Read the model definition and answer for the solid it produces. Units are mm, in the model's axes. Face numbers are marked on the shaded views. A direction names the side the tool comes from. Coordinates: 2 decimals unless noted, no trailing zeros. Write each loop counter-clockwise with the first axis right and the second up, starting at its lowest first coordinate (ties: lowest second). Pieces come first, ordered by that corner, then holes.
1) The part is cut by section C-C (y = 20.5). Determine the outline of the cut face in (x, z), then the cut area to 3 significant figures.
2) The part is cut by section D-D (x = 14). Determine the outline of the cut face in (y, z).
3) Each of these flat-tipped pins is pushed along its axis until it touches: pin 1 Ø0.7 at (y, z) = (40.5, 13) entering from +X; pin 2 Ø0.5 at (x, z) = (-20, 5) entering from +Y; pin 3 Ø3.5 at (x, z) = (1, -8) entering from -Y. Where does it stop, or does it pass through?
4) Find the intervals of material crossed by line 1 (X direction, y = 37, z = 20); line 2 (Z direction, x = -14.5, y = 7.5); line 3 (X direction, y = 20, z = 20.5), in increasing order.
5) Which of the six approach directions +Z, -Z, +X, -X, +Y, -Y give full straight-line access (tool end or side, diameter ignored) to the marked faces 1, 2, 3, 4 and 5?
6) The part is cut by section A-A (x = 0). Determine the outline of the cut face in (y, z).
7) Determine the mould class of the marked faces 6, 7 and 8 for opening direction X: +X half, -X half, draft (parallel to the pull), parting line (faces both ways), or undercut.
8) The part is cut by section B-B (z = 3.5). Determine the outline of the cut face in (x, y).
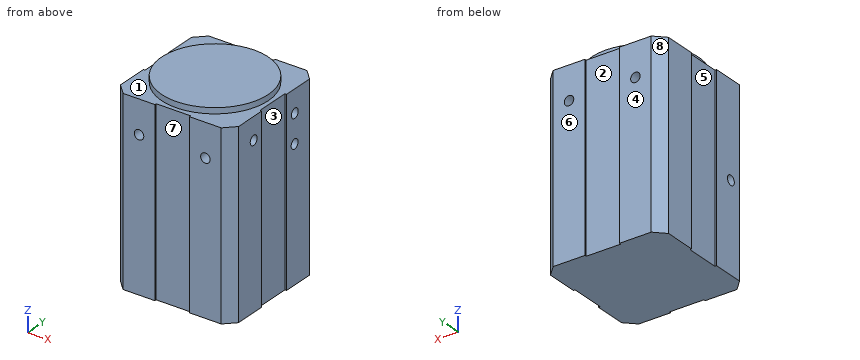
from build123d import *

# Parameters (mm, degrees)
SKETCH_1_W                       = 41
SKETCH_1_H                       = 63
EXTRUDE_1_DEPTH                  = 41
HOLE_WIZARD_M4_1_AT_2_COUNT      = 2
HOLE_WIZARD_M4_1_AT_2_PITCH      = 23
CHAMFER_1_SIZE                   = 3.5
CUT_EXTRUDE_1_REACH              = 79.912
SKETCH_4_W                       = 12
SKETCH_4_H                       = 0.6
SKETCH_4_W_2                     = 0.6
SKETCH_4_H_2                     = 12
SKETCH_5_R                       = 18.5
EXTRUDE_2_DEPTH                  = 2
HOLE_WIZARD_M4_3_D               = 3.3
HOLE_WIZARD_M4_3_DEPTH           = 10.1
HOLE_WIZARD_M4_3_TIP             = 0.991420021
HOLE_WIZARD_M4_3_ON_FACE_2_D     = 3.3
HOLE_WIZARD_M4_3_ON_FACE_2_DEPTH = 10.1
HOLE_WIZARD_M4_3_ON_FACE_2_TIP   = 0.991420021


with BuildPart() as part:
    # 草图1 → 凸台-拉伸1 (new body)
    with BuildSketch(Plane(origin=(0, 0, 0), x_dir=(1, 0, 0), z_dir=(0, 1, 0))):
        Rectangle(SKETCH_1_W, SKETCH_1_H)
    extrude(amount=EXTRUDE_1_DEPTH)

    # 草图3 → M4 螺纹孔1 (revolve, cut)
    with BuildSketch(Plane(origin=(-11.5, 41, 20), x_dir=(0, 0, 1), z_dir=(1, 0, 0))):
        Polygon((0, 0), (0, 6.991420021), (1.65, 6), (1.65, 0), align=None)
    hole_wizard_m4_1 = revolve(axis=Axis((-11.5, 47.35, 20), (0, -1, 0)), mode=Mode.SUBTRACT)

    # M4 螺纹孔1 at 2: M4 螺纹孔1 ×2
    with Locations(*[(i * HOLE_WIZARD_M4_1_AT_2_PITCH, 0, 0) for i in range(1, HOLE_WIZARD_M4_1_AT_2_COUNT)]):
        add(hole_wizard_m4_1, mode=Mode.SUBTRACT)

    # 镜向1: M4 螺纹孔1 across plane
    add(hole_wizard_m4_1.mirror(Plane.ZX.offset(20.5)), mode=Mode.SUBTRACT)

    # 镜向1 copy 1 sketch → 镜向1 copy 1 (revolve, cut)
    with BuildSketch(Plane(origin=(11.5, 0, 20), x_dir=(0, 0, 1), z_dir=(1, 0, 0))):
        Polygon((0, 0), (0, -6.991420021), (1.65, -6), (1.65, 0), align=None)
    revolve(axis=Axis((11.5, -6.35, 20), (0, -1, 0)), mode=Mode.SUBTRACT)

    # 倒角1
    chamfer_1_edges = [part.edges().sort_by_distance(p)[0] for p in [
        (-20.5, 41, 0),
        (20.5, 41, 0),
        (-20.5, 0, 0),
        (20.5, 0, 0),
    ]]
    chamfer(chamfer_1_edges, length=CHAMFER_1_SIZE)

    # 草图4 → 切除-拉伸1 (cut, up to next)
    with BuildSketch(Plane.XY.offset(31.5), mode=Mode.PRIVATE) as cut_extrude_1_sk1:
        with Locations((0, 40.7)):
            Rectangle(SKETCH_4_W, SKETCH_4_H)
    cut_extrude_1_tool1 = extrude(cut_extrude_1_sk1.sketch, amount=-CUT_EXTRUDE_1_REACH, mode=Mode.PRIVATE) & part.part
    # 草图4 → 切除-拉伸1 (cut, up to next)
    with BuildSketch(Plane.XY.offset(31.5), mode=Mode.PRIVATE) as cut_extrude_1_sk2:
        with Locations((20.2, 20.5)):
            Rectangle(SKETCH_4_W_2, SKETCH_4_H_2)
    cut_extrude_1_tool2 = extrude(cut_extrude_1_sk2.sketch, amount=-CUT_EXTRUDE_1_REACH, mode=Mode.PRIVATE) & part.part
    # 草图4 → 切除-拉伸1 (cut, up to next)
    with BuildSketch(Plane.XY.offset(31.5), mode=Mode.PRIVATE) as cut_extrude_1_sk3:
        with Locations((0, 0.3)):
            Rectangle(SKETCH_4_W, SKETCH_4_H)
    cut_extrude_1_tool3 = extrude(cut_extrude_1_sk3.sketch, amount=-CUT_EXTRUDE_1_REACH, mode=Mode.PRIVATE) & part.part
    # 草图4 → 切除-拉伸1 (cut, up to next)
    with BuildSketch(Plane.XY.offset(31.5), mode=Mode.PRIVATE) as cut_extrude_1_sk4:
        with Locations((-20.2, 20.5)):
            Rectangle(SKETCH_4_W_2, SKETCH_4_H_2)
    cut_extrude_1_tool4 = extrude(cut_extrude_1_sk4.sketch, amount=-CUT_EXTRUDE_1_REACH, mode=Mode.PRIVATE) & part.part
    add(cut_extrude_1_tool1.solids().sort_by_distance((0, 40.7, 31.5))[0], mode=Mode.SUBTRACT)
    add(cut_extrude_1_tool2.solids().sort_by_distance((20.2, 20.5, 31.5))[0], mode=Mode.SUBTRACT)
    add(cut_extrude_1_tool3.solids().sort_by_distance((0, 0.3, 31.5))[0], mode=Mode.SUBTRACT)
    add(cut_extrude_1_tool4.solids().sort_by_distance((-20.2, 20.5, 31.5))[0], mode=Mode.SUBTRACT)

    # 草图5 → 凸台-拉伸2 (add)
    with BuildSketch(Plane.XY.offset(31.5)):
        with Locations((0, 20.5)):
            Circle(SKETCH_5_R)
    extrude(amount=EXTRUDE_2_DEPTH)

    # M4 螺纹孔3
    with Locations(Plane(origin=(20.5, 30.405354364, 23.651006077), x_dir=(0, 0, 1), z_dir=(1, 0, 0))):
        with Locations((0, 0), (-9.799993904, 0.098891397), (0.188566307, 19.700944215)):
            Hole(HOLE_WIZARD_M4_3_D / 2, depth=HOLE_WIZARD_M4_3_DEPTH)
            with Locations((0, 0, -(HOLE_WIZARD_M4_3_DEPTH + HOLE_WIZARD_M4_3_TIP / 2))):  # 118° drill point
                Cone(0, HOLE_WIZARD_M4_3_D / 2, HOLE_WIZARD_M4_3_TIP, mode=Mode.SUBTRACT)

    # M4 螺纹孔3 on face 2
    with Locations(Plane(origin=(-20.5, 7.687513873, -0.982360161), x_dir=(0, 0, -1), z_dir=(-1, 0, 0))):
        with Locations((0, 0)):
            Hole(HOLE_WIZARD_M4_3_ON_FACE_2_D / 2, depth=HOLE_WIZARD_M4_3_ON_FACE_2_DEPTH)
            with Locations((0, 0, -(HOLE_WIZARD_M4_3_ON_FACE_2_DEPTH + HOLE_WIZARD_M4_3_ON_FACE_2_TIP / 2))):  # 118° drill point
                Cone(0, HOLE_WIZARD_M4_3_ON_FACE_2_D / 2, HOLE_WIZARD_M4_3_ON_FACE_2_TIP, mode=Mode.SUBTRACT)


solid = part.part
Reported:
1. outline: (-19.9, -31.5) - (19.9, -31.5) - (19.9, 31.5) - (18.5, 31.5) - (18.5, 33.5) - (-18.5, 33.5) - (-18.5, 31.5) - (-19.9, 31.5) - close
1. area: 2,580 mm2
2. outline: (0, -31.5) - (41, -31.5) - (41, 31.5) - (32.59, 31.5) - (32.59, 33.5) - (8.41, 33.5) - (8.41, 31.5) - (0, 31.5) - close; hole circle Ø3.3 at (10.7, 23.84); hole circle Ø3.3 at (30.31, 13.85); hole circle Ø3.3 at (30.41, 23.65)
3. pin 1: stops at x = 17.85
3. pin 2: stops at y = 38.25
3. pin 3: stops at y = 0.6
4. line 1: x = -20.5 to -13.15, -9.85 to 9.85, 13.15 to 20.5
4. line 2: z = -31.5 to -2.62, 0.66 to 31.5
4. line 3: x = -19.9 to 19.9
5. face 1: +Z
5. face 2: +Z, -Z, +Y
5. face 3: +Z, -Z, +X
5. face 4: +Z, -Z, +X, -X, +Y
5. face 5: +Z, -Z, -X
6. outline: (0.6, -31.5) - (40.4, -31.5) - (40.4, 31.5) - (39, 31.5) - (39, 33.5) - (2, 33.5) - (2, 31.5) - (0.6, 31.5) - close
7. face 6: draft
7. face 7: undercut
7. face 8: -X half
8. outline: (-20.5, 3.5) - (-17, 0) - (-6, 0) - (-6, 0.6) - (6, 0.6) - (6, 0) - (17, 0) - (20.5, 3.5) - (20.5, 14.5) - (19.9, 14.5) - (19.9, 26.5) - (20.5, 26.5) - (20.5, 37.5) - (17, 41) - (6, 41) - (6, 40.4) - (-6, 40.4) - (-6, 41) - (-17, 41) - (-20.5, 37.5) - (-20.5, 26.5) - (-19.9, 26.5) - (-19.9, 14.5) - (-20.5, 14.5) - close
